from build123d import *

# Parameters (mm, degrees)
CROQUIS2_W              = 63.5
CROQUIS2_H              = 130
SALIENTE_EXTRUIR1_DEPTH = 6.31
CROQUIS3_W              = 63.5
CROQUIS3_H              = 6.31
SALIENTE_EXTRUIR2_DEPTH = 513.44
CROQUIS4_W              = 63.5
CROQUIS4_H              = 6.31
SALIENTE_EXTRUIR3_DEPTH = 1787.3
CROQUIS9_W              = 63.5
CROQUIS9_H              = 6.31
SALIENTE_EXTRUIR4_DEPTH = 98
CROQUIS12_R             = 5
CORTAR_EXTRUIR1_DEPTH   = 10


with BuildPart() as part:
    # Croquis2 → Saliente-Extruir1 (new body)
    with BuildSketch(Plane.XY):
        Rectangle(CROQUIS2_W, CROQUIS2_H)
    extrude(amount=SALIENTE_EXTRUIR1_DEPTH)

    # Croquis3 → Saliente-Extruir2 (add)
    with BuildSketch(Plane.XY.offset(6.31)):
        with Locations((0, -61.845)):
            Rectangle(CROQUIS3_W, CROQUIS3_H)
    extrude(amount=SALIENTE_EXTRUIR2_DEPTH)

    # Croquis4 → Saliente-Extruir3 (add)
    with BuildSketch(Plane(origin=(31.75, 0, 0), x_dir=(0, 0, -1), z_dir=(1, 0, 0))):
        with Locations((-488, -61.845)):
            Rectangle(CROQUIS4_W, CROQUIS4_H)
    extrude(amount=SALIENTE_EXTRUIR3_DEPTH)

    # Barrer2: sweep along a curve in space
    with BuildLine() as barrer2_path:
        Line((1787.3, -61.845, 519.75), (1787.3, -61.845, 546.16))
        Line((1787.3, -61.845, 546.16), (1787.3, 69.915, 546.16))
        Line((1787.3, 69.915, 546.16), (1787.3, 69.915, 1340.16))
    # Croquis9 → Barrer2 (sweep)
    with BuildSketch(Plane.XY.offset(519.75)):
        with Locations((1787.3, -61.845)):
            Rectangle(CROQUIS9_W, CROQUIS9_H)
    sweep(path=barrer2_path.line, transition=Transition.RIGHT)

    # Croquis11 → Saliente-Extruir4 (add)
    with BuildSketch(Plane.ZY.offset(31.75)):
        Polygon((0, 65), (-35.006192049, 134.080780284), (-29.377619212, 136.933019371), (6.31, 65), align=None)
    extrude(amount=-SALIENTE_EXTRUIR4_DEPTH)

    # Croquis12 → Cortar-Extruir1 (cut)
    with BuildSketch(Plane(origin=(0, 73.07, 0), x_dir=(1, 0, 0), z_dir=(0, 1, 0))):
        with Locations(Location((1787.3, -1307.16, 0), (0, 0, 270))):
            Circle(CROQUIS12_R)
        with Locations(Location((1787.3, -1087.16, 0), (0, 0, 270))):
            Circle(CROQUIS12_R)
    extrude(amount=-CORTAR_EXTRUIR1_DEPTH, mode=Mode.SUBTRACT)


solid = part.part
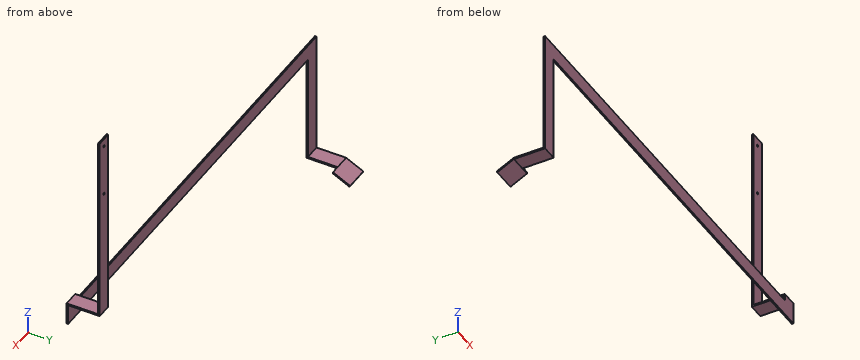
Work out the finished part from the listing and answer in its coordinate system (mm). Round coordinates to 2 decimals unless told otherwise and drop trailing zeros. Order: outer loops, then holes, each group sorted by start corner. A loop starts at its lowest first (then second) coordinate and runs counter-clockwise, first axis right, second up. Notation, with made-up numbers: M 76,43 L 94,43 A19 ccw 94,73 Z; hole C 42,-8 d6. An arc over 180 degrees is marked long. Put each result on its own line as item: value. Start each with the question number.
Q1. Flat-ended cylindrical pins translate along their axes: pin 1 (3 mm diameter, centred on x = 54.5, z = 3, fed in from -Y); pin 2 (13 mm diameter, centred on x = 1787.3, z = 1087.16, fed in from -Y); pin 3 (5 mm diameter, centred on x = 508.5, y = -63.5, fed in from +Z). Find the tip coordinate at first contact, or state that the pin passes through.
Q2. Section A-A, the plane y = -14 is taken. Write down the section's boundary in (x, z) (3 decimals).
Q3. Straight lines are drawn through the part: L1, parallel to Z at x = 1787.3, y = 71.25 (3 decimals); L2, parallel to X at y = 70, z = 1087; L3, parallel to X at y = 73, z = 980.5. For each, find the intervals that lie inside material, in ascending order. Write a range as [from, to].
Q4. Section C-C, the plane z = 1017 is taken. Write down the section's boundary in (x, y).
Q5. Section B-B, the plane x = 1047.5 is taken. Write down the section's boundary in (y, z), and give its area (3 significant figures).
Findings below:
1. pin 1: stops at y = 65
1. pin 2: stops at y = 66.76
1. pin 3: stops at z = 519.75
2. outline: M -31.75,0 L 31.75,0 L 31.75,6.31 L -31.75,6.31 Z; M 1755.55,543.005 L 1819.05,543.005 L 1819.05,549.315 L 1755.55,549.315 Z
3. L1: z = [543.005, 1082.16], [1092.16, 1302.16], [1312.16, 1340.16]
3. L2: x = [1755.55, 1782.3], [1792.3, 1819.05]
3. L3: x = [1755.55, 1819.05]
4. outline: M 1755.55,66.76 L 1819.05,66.76 L 1819.05,73.07 L 1755.55,73.07 Z
5. outline: M -65,456.25 L -58.69,456.25 L -58.69,519.75 L -65,519.75 Z
5. area: 401 mm^2
